Could you check a few things on this model? Use its own coordinates, in mm. A direction names the side the tool comes from. Coordinates: 2 decimals unless noted, no trailing zeros. Loops run counter-clockwise (first coordinate to the right, second up) from the corner with the lowest first, then second, coordinate; pieces in that order, holes last. Notation, with made-up numbers: (23, 84.5) - (41, 84.5) arc R24 ccw to (41, 120.5) - close; hole circle Ø4 at (83, -22). An arc over 180 degrees is marked (long way). Use CSV: the item, a comma, the result in double quotes.
from build123d import *

# Parameters (mm, degrees)
SKETCH10_W                  = 2.54
SKETCH10_H                  = 2.54
BOSS_EXTRUDE3_DEPTH         = 152.4
BOSS_EXTRUDE4_DEPTH         = 177.8
SKETCH14_W                  = 25.4
SKETCH14_H                  = 25.4
CUT_EXTRUDE1_DEPTH          = 184.407350223
F_1_4_0_25_DIAMETER_HOLE1_D = 6.35
F_1_4_0_25_DIAMETER_HOLE2_D = 6.35


with BuildPart() as part:
    # Sketch10 → Boss-Extrude3 (new body)
    with BuildSketch(Plane(origin=(0, 0, 0), x_dir=(0, 0, -1), z_dir=(1, 0, 0))):
        with BuildLine():
            Line((-2.54, 5.08), (0, 5.08))
            Line((0, 5.08), (0, 10.16))
            Line((0, 10.16), (-2.54, 10.16))
            Line((-2.54, 10.16), (-6.35, 10.16))
            ThreePointArc((-6.35, 10.16), (-6.580814495, 10.012022021), (-6.542688341, 9.740509205))
            Line((-6.542688341, 9.740509205), (-2.54, 5.08))
        make_face()
        with Locations((-1.27, 11.43)):
            Rectangle(SKETCH10_W, SKETCH10_H)
        with BuildLine():
            Line((0, 10.16), (0, 5.08))
            Line((0, 5.08), (2.54, 5.08))
            Line((2.54, 5.08), (6.542688341, 9.740509205))
            ThreePointArc((6.542688341, 9.740509205), (6.580814495, 10.012022021), (6.35, 10.16))
            Line((6.35, 10.16), (2.54, 10.16))
            Line((2.54, 10.16), (0, 10.16))
        make_face()
        with Locations((1.27, 11.43)):
            Rectangle(SKETCH10_W, SKETCH10_H)
    extrude(amount=-BOSS_EXTRUDE3_DEPTH)

    # Sketch11 → Boss-Extrude4 (add)
    with BuildSketch(Plane(origin=(0, 0, 0), x_dir=(0, 0, -1), z_dir=(1, 0, 0))):
        Polygon((6.35, 12.7), (-6.35, 12.7), (-6.35, 43.1), (-1.5875, 43.1), (-1.5875, 17.7), (1.5875, 17.7), (1.5875, 43.1), (6.35, 43.1), align=None)
    extrude(amount=-BOSS_EXTRUDE4_DEPTH)

    # Sketch14 → Cut-Extrude1 (cut, through all)
    with BuildSketch(Plane(origin=(0, 0, -6.35), x_dir=(-1, 0, 0), z_dir=(0, 0, -1))):
        with Locations((165.1, 30.4)):
            Rectangle(SKETCH14_W, SKETCH14_H)
    extrude(amount=-CUT_EXTRUDE1_DEPTH, mode=Mode.SUBTRACT)

    # 1/4 (0.25) Diameter Hole1 (through all)
    with Locations(Plane(origin=(0, 0, -6.35), x_dir=(-1, 0, 0), z_dir=(0, 0, -1))):
        with Locations((139.7, 27.9), (12.7, 27.9), (76.2, 27.9)):
            Hole(F_1_4_0_25_DIAMETER_HOLE1_D / 2)

    # 1/4 (0.25) Diameter Hole2 (through all)
    with Locations(Plane(origin=(0, 17.7, 0), x_dir=(1, 0, 0), z_dir=(0, 1, 0))):
        with Locations((-165.1, 0)):
            Hole(F_1_4_0_25_DIAMETER_HOLE2_D / 2)


solid = part.part
(1) Please list where these lines run through material, in increasing order: line 1 (Y direction, x = -12.7, z = -3.6) (3 decimals); line 2 (Z direction, x = -126.5, y = 32.5); line 3 (Y direction, x = -139.7, z = -2.8) (3 decimals).
Computed:
line 1,"y = 6.314 to 10.16, 12.7 to 24.725, 31.075 to 43.1"
line 2,"z = -6.35 to -1.59, 1.59 to 6.35"
line 3,"y = 5.383 to 10.16, 12.7 to 24.725, 31.075 to 43.1"
(2) Will these pins go through, and if not, where does the flat tip stop? pin 1 (15 mm diameter, centred on x = -78.5, y = 30.5, fed in from +Z); pin 2 (4 mm diameter, centred on x = -76.2, y = 27.9, fed in from +Z) (3 decimals); pin 3 (12.5 mm diameter, centred on x = -47.5, y = 36.5, fed in from -Z); pin 4 (1 mm diameter, centred on x = -22.5, y = 12, fed in from -Z).
Computed:
pin 1,"stops at z = 6.35"
pin 2,"passes through"
pin 3,"stops at z = -6.35"
pin 4,"stops at z = -2.54"
(3) Which directions (+Z, -Z, +X, -X, +Y, -Y) give clear straight access to the entire face, cutting with the end or side of a thin tool? Please do faces 1 (the face through (-75, 10.16, 4)), 2 (the face through (-152.4, 30, 4)), 3 (the face through (-75, 10.16, -4)), 4 (the face through (-88, 28, -6.35)).
Computed:
face 1,"+Z, +X, -X"
face 2,"+Z, -Z, -X, +Y"
face 3,"-Z, +X, -X"
face 4,"-Z, +X, -X, +Y"
(4) Suppose I cut it at C-C (z = 0). Write out the boundary of the cut face in (x, y) (3 decimals), plus the area to 3 significant figures.
Computed:
outline,"(-177.8, 12.7) - (-168.275, 12.7) - (-168.275, 17.7) - (-177.8, 17.7) - close; (-161.925, 12.7) - (-152.4, 12.7) - (-152.4, 5.08) - (0, 5.08) - (0, 17.7) - (-161.925, 17.7) - close"
area,"2,020 mm²"
(5) Suppose I cut it at A-A (y = 27.9). State how many separate pieces and enclosed holes the cut face has, plus the area to 3 significant figures.
Computed:
separate pieces,"8"
enclosed holes,"0"
area,"1,270 mm²"
(6) Suppose I cut it at B-B (x = -165.1). Write out the boundary of the cut face in (y, z) (3 decimals), plus the area to 4 significant figures.
Computed:
outline,"(12.7, -6.35) - (17.7, -6.35) - (17.7, -3.175) - (12.7, -3.175) - close; (12.7, 3.175) - (17.7, 3.175) - (17.7, 6.35) - (12.7, 6.35) - close"
area,"31.75 mm²"
(7) Suppose I cut it at D-D (y = 20). Write out the boundary of the cut face in (x, z).
Computed:
outline,"(-152.4, -6.35) - (0, -6.35) - (0, -1.59) - (-152.4, -1.59) - close; (-152.4, 1.59) - (0, 1.59) - (0, 6.35) - (-152.4, 6.35) - close"
(8) Thinking about a two-plate mould opening in X: for faces 5 (the face through (-152.4, 9, 0)), 6 (the face through (-13.11, 31.05, -3.94)), 7 (the face through (-75, 33, -1.588)), which applies, +X half, -X half, draft (parallel to the pull), parting line (faces both ways), or undercut?
Computed:
face 5,"-X half"
face 6,"undercut"
face 7,"draft"
